The model under review builds one solid part; all positions refer to its coordinate system, in mm. Give positions to 0.01 mm unless a question says otherwise; leave off trailing zeros. Loops run counter-clockwise (first coordinate to the right, second up) from the corner with the lowest first, then second, coordinate; pieces in that order, holes last. Notation, with made-up numbers: M -19,-32.75 L 2,-32.75 A32 ccw 2,-0.75 Z; hole C -18.5,61.5 d9. An arc over 180 degrees is marked long. Put each result on its own line as item: value. Start each with the question number.
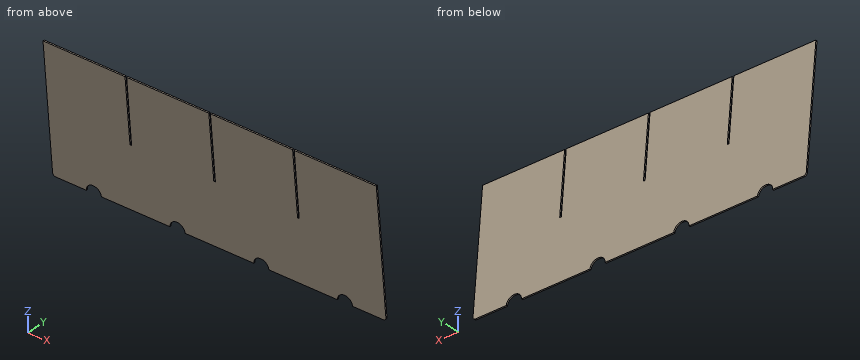
```python
from build123d import *

# Parameters (mm, degrees)
EXTRUDE_1_DEPTH = 1


with BuildPart() as part:
    # 草图1 → 凸台-拉伸1 (new body)
    with BuildSketch(Plane(origin=(0, 53.933062278, 5.010311528), x_dir=(-1, 0, 0), z_dir=(5.133494296529154e-15, 0.9957126460708378, 0.09250041326724258))):
        with BuildLine():
            Line((-121.5, 905.593751703), (-121.5, 812.593751703))
            ThreePointArc((-121.5, 812.593751703), (-120.914213563, 811.179538141), (-119.5, 810.593751703))
            Line((-119.5, 810.593751703), (-97.1, 810.593751703))
            ThreePointArc((-97.1, 810.593751703), (-91.6, 816.093751703), (-86.1, 810.593751703))
            Line((-86.1, 810.593751703), (-36.05, 810.593751703))
            ThreePointArc((-36.05, 810.593751703), (-30.55, 816.093751703), (-25.05, 810.593751703))
            Line((-25.05, 810.593751703), (25.05, 810.593751703))
            ThreePointArc((25.05, 810.593751703), (30.55, 816.093751703), (36.05, 810.593751703))
            Line((36.05, 810.593751703), (86.1, 810.593751703))
            ThreePointArc((86.1, 810.593751703), (91.6, 816.093751703), (97.1, 810.593751703))
            Line((97.1, 810.593751703), (119.5, 810.593751703))
            ThreePointArc((119.5, 810.593751703), (120.914213562, 811.179538141), (121.5, 812.593751703))
            Line((121.5, 812.593751703), (121.5, 905.593751703))
            Line((121.5, 905.593751703), (61.7, 905.593751703))
            Line((61.7, 905.593751703), (61.7, 857.583834348))
            Line((61.7, 857.583834348), (60.5, 857.593751703))
            Line((60.5, 857.593751703), (60.5, 905.593751703))
            Line((60.5, 905.593751703), (0.6, 905.593751703))
            Line((0.6, 905.593751703), (0.6, 857.593751703))
            Line((0.6, 857.593751703), (-0.6, 857.593751703))
            Line((-0.6, 857.593751703), (-0.6, 905.593751703))
            Line((-0.6, 905.593751703), (-60.5, 905.593751703))
            Line((-60.5, 905.593751703), (-60.5, 857.603476177))
            Line((-60.5, 857.603476177), (-61.7, 857.593751703))
            Line((-61.7, 857.593751703), (-61.7, 905.593751703))
            Line((-61.7, 905.593751703), (-121.5, 905.593751703))
        make_face()
    extrude(amount=-EXTRUDE_1_DEPTH)


solid = part.part
```
Item 1: Consider section B-B, the plane x = -20.5. Write out the cut boundary in (y, z), plus the area to 3 significant figures.
Item 2: Clearance check with flat-ended pins moving along their axes: pin 1 Ø1.5 at (x, z) = (38.5, 884.5) entering from +Y; pin 2 Ø12 at (x, z) = (-88.5, 866) entering from +Y; pin 3 Ø2.5 at (y, z) = (-27.5, 885.5) entering from +X; pin 4 Ø12 at (x, z) = (38, 857) entering from +Y. State where each tip first meets the part, or that it passes through.
Item 3: Consider section C-C, the plane z = 853.5. Write out the cut boundary in (x, y).
Item 4: To check wall thickness, follow L1, parallel to Y at x = 24, z = 854; L2, parallel to Y at x = -92.5, z = 888. State the ranges of each line that lie inside material, in increasing order. Write a range as [from, to].
Item 5: Consider section A-A, the plane z = 871.5. Write out the cut boundary in (x, y).
Report:
1. outline: M -30.83,906.63 L -22.04,812.04 L -21.05,812.13 L -29.83,906.72 Z
1. area: 95.0 mm²
2. pin 1: y = -27.7
2. pin 2: y = -25.49
2. pin 3: x = 121.5
2. pin 4: y = -24.66
3. outline: M -121.5,-25.89 L 121.5,-25.89 L 121.5,-24.89 L -121.5,-24.89 Z
4. L1: [-25.94, -24.94]
4. L2: [-29.1, -28.1]
5. outline: M -121.5,-27.57 L -61.7,-27.57 L -61.7,-26.56 L -121.5,-26.56 Z; M -60.5,-27.57 L -0.6,-27.57 L -0.6,-26.56 L -60.5,-26.56 Z; M 0.6,-27.57 L 60.5,-27.57 L 60.5,-26.56 L 0.6,-26.56 Z; M 61.7,-27.57 L 121.5,-27.57 L 121.5,-26.56 L 61.7,-26.56 Z
